Can you work these out from the model? Positions are in its coordinate system, mm. A direction names the side the tool comes from. Give positions to 0.01 mm unless a question says otherwise; leave off trailing zeros. Order: outer loops, then holes, each group sorted by start corner. A loop starts at its lowest first (then second) coordinate and runs counter-clockwise, first axis right, second up. Notation, with made-up numbers: M 23.25,-27.75 L 35.25,-27.75 A20 ccw 35.25,-14.75 Z; hole C -40,72 d11. An arc over 180 degrees is marked long. One line per question, with ' | ' between items. Start each with the question number.
1) If we section it at C-C, the plane z = 9: Please give me the cut outline in (x, y).
2) I'm going to push flat-ended pins straight in: pin 1 Ø1.5 at (x, z) = (13, -16) entering from +Y; pin 2 Ø5 at (x, y) = (17.5, -32) entering from +Z; pin 3 Ø1.8 at (x, y) = (-18.5, -23) entering from +Z. Where does each tip first touch, or does it pass through?
3) Thinking about a two-plate mould opening in X: for faces 1 (the flat face through (-15.15, 14, -48)), 2 (the flat face through (18, -34, -70.15)), which applies, +X half, -X half, draft (parallel to the pull), parting line (faces both ways), or undercut?
4) If we section it at D-D, the plane y = -55: Please give me the cut outline in (x, z), plus the area to 3 significant figures.
5) For faces 3 (the flat face through (0, 28, -48)), 4 (the flat face through (0, -5, -13)), 5 (the flat face through (0, 32, -21.15)), 6 (the flat face through (0, 0, -27)), 7 (the flat face through (-0.21, -12.7, -35.25)), which set-ups out of +Z, -Z, +X, -X, +Y, -Y let a thin tool reach every point of the face, with its end or its side?
6) If we section it at A-A, the plane z = -15.5: Please give me the cut outline in (x, y), plus the area to 4 significant figures.
7) If we section it at B-B, the plane x = 0: Please give me the cut outline in (y, z), plus the area to 3 significant figures.
8) Please list where these lines run through material, in increasing order: line 1 along X through (y, z) = (-2.75, -15.5); line 2 along Z through (x, y) = (-15.5, -1.4); line 3 along X through (y, z) = (-53, -63). Write a range as [from, to].
```python
from build123d import *

# Parameters (mm, degrees)
F0_W      = 42.3
F0_H      = 42.3
F0_R      = 12.5
F1_DEPTH  = 5
F2_D      = 3.1
F0_H_2    = 5
F3_DEPTH  = 5
F4_DEPTH  = 34
F5_W      = 30.3
F5_H      = 28
F6_DEPTH  = 5
F7_DEPTH  = 50
F9_DEPTH  = 42.3
F10_W     = 30.3
F10_H     = 56.616878205
F11_DEPTH = 25
F12_W     = 30.3
F12_H     = 46.3778315229
F13_DEPTH = 25


with BuildPart() as f1:
    # F0 (on Front) → F1 (new body)
    with BuildSketch(Plane.XZ):
        Rectangle(F0_W, F0_H)
        Circle(F0_R, mode=Mode.SUBTRACT)
    extrude(amount=F1_DEPTH)

    # F2 (through all)
    with Locations(Plane(origin=(0, 0, 0), x_dir=(1, 0, 0), z_dir=(0, 1, 0))):
        with Locations((-15.5, -15.5), (-15.5, 15.5), (15.5, 15.5), (15.5, -15.5)):
            Hole(F2_D / 2)

    # F0 (on Front) → F3 (join)
    with BuildSketch(Plane.XZ):
        with Locations((0, -23.65)):
            Rectangle(F0_W, F0_H_2)
    extrude(amount=F3_DEPTH)

    # F0 (on Front) → F4 (join)
    with BuildSketch(Plane.XZ):
        with Locations((0, -23.65)):
            Rectangle(F0_W, F0_H_2)
    extrude(amount=-F4_DEPTH)

    # F5 (on face) → F6 (cut)
    with BuildSketch(Plane.XY.offset(-21.15)):
        with Locations((0, 14)):
            Rectangle(F5_W, F5_H)
    extrude(amount=-F6_DEPTH, mode=Mode.SUBTRACT)

    # F7 (add): a face of the model
    f7_faces = [f1.faces().sort_by_distance(p)[0] for p in [
        (0, -4.4246488029, -26.15),
    ]]
    extrude(f7_faces, amount=F7_DEPTH)

    # F8 (on face) → F9 (join)
    with BuildSketch(Plane.YZ.offset(21.15)):
        Polygon((-76.4074003371, -76.15), (-5, -76.15), (-5, -26.15), align=None)
        Polygon((-57.3778315229, -70.15), (-11, -37.6758927618), (-11, -70.15), align=None, mode=Mode.SUBTRACT)
    extrude(amount=-F9_DEPTH)

    # F10 (on face) → F11 (cut)
    with BuildSketch(Plane(origin=(0, 14.0829899932, -20.1125940878), x_dir=(1, 0, 0), z_dir=(0, 0.5735764364, -0.8191520443))):
        with Locations((0, 58.9291158964)):
            Rectangle(F10_W, F10_H)
    extrude(amount=-F11_DEPTH, mode=Mode.SUBTRACT)

    # F12 (on face) → F13 (cut)
    with BuildSketch(Plane.XY.offset(-70.15)):
        with Locations((0, -34.1889157615)):
            Rectangle(F12_W, F12_H)
    extrude(amount=-F13_DEPTH, mode=Mode.SUBTRACT)


solid = f1.part
```
Results found:
1) outline: M -21.15,-5 L -8.67,-5 L -8.67,0 L -21.15,0 Z; M 8.67,-5 L 21.15,-5 L 21.15,0 L 8.67,0 Z
2) pin 1: stops at y = 0 | pin 2: stops at z = -43.31 | pin 3: stops at z = -38.12
3) face 1: undercut | face 2: draft
4) outline: M -21.15,-76.15 L -15.15,-76.15 L -15.15,-70.15 L -21.15,-70.15 Z; M -21.15,-68.49 L -15.15,-68.49 L -15.15,-61.16 L -21.15,-61.16 Z; M 15.15,-76.15 L 21.15,-76.15 L 21.15,-70.15 L 15.15,-70.15 Z; M 15.15,-68.49 L 21.15,-68.49 L 21.15,-61.16 L 15.15,-61.16 Z | area: 160 mm²
5) face 3: +Z, -Z | face 4: +Z, +X, -X, -Y | face 5: +Z, +X, -X, +Y | face 6: +Z | face 7: -Z, -Y
6) outline: M -21.15,-5 L -17.05,-5 L -17.05,0 L -21.15,0 Z; M -13.95,-5 L 13.95,-5 L 13.95,0 L -13.95,0 Z; M 17.05,-5 L 21.15,-5 L 21.15,0 L 17.05,0 Z | area: 180.5 mm²
7) outline: M -76.41,-76.15 L -57.38,-76.15 L -57.38,-70.15 L -60.82,-65.24 Z; M -14.44,-32.76 L -11,-37.68 L -11,-76.15 L 0,-76.15 L 0,-12.5 L -5,-12.5 L -5,-26.15 Z; M -5,12.5 L 0,12.5 L 0,21.15 L -5,21.15 Z; M 28,-76.15 L 34,-76.15 L 34,-21.15 L 28,-21.15 Z | area: 1,110 mm²
8) line 1: x = [-21.15, -17.05], [-13.95, 13.95], [17.05, 21.15] | line 2: z = [-76.15, -17.05], [-13.95, 13.95], [17.05, 21.15] | line 3: x = [-21.15, -15.15], [15.15, 21.15]
